from build123d import *

# Parameters (mm, degrees)
SKETCH2_R          = 1
CUT_EXTRUDE1_DEPTH = 52.147287318


with BuildPart() as part:
    # Sketch1 → Revolve1 (revolve)
    with BuildSketch(Plane.XY, mode=Mode.PRIVATE) as revolve1_sk:
        Polygon((32.65, -4.5), (10, -4.5), (10, -17.5), (7, -17.5), (7, 4.5), (32.65, 4.5), (32.65, 1.5), (28.65, 1.5), (28.65, -1.5), (32.65, -1.5), align=None)
    revolve(revolve1_sk.sketch.rotate(Axis((0, 0, 0), (0, 1, 0)), 90), axis=Axis((0, 0, 0), (0, 1, 0)))

    # Sketch2 → Cut-Extrude1 (cut, through all)
    with BuildSketch(Plane(origin=(0, 4.5, 0), x_dir=(1, 0, 0), z_dir=(0, 1, 0))):
        with Locations(Location((23.65, 0, 0), (0, 0, 270))):
            Circle(SKETCH2_R)
    extrude(amount=-CUT_EXTRUDE1_DEPTH, mode=Mode.SUBTRACT)


solid = part.part
The model under review builds one solid part; all positions refer to its coordinate system, in mm. A direction names the side the tool comes from. Coordinates: 2 decimals unless noted, no trailing zeros. Order: outer loops, then holes, each group sorted by start corner. A loop starts at its lowest first (then second) coordinate and runs counter-clockwise, first axis right, second up. Notation, with made-up numbers: (-8, 70.25) -> (48, 70.25) arc R37 ccw to (48, 106.25) -> close; hole circle Ø1 at (-39.75, 1). An arc over 180 degrees is marked (long way). Answer in a Markdown table with one row per item.
(1) Consider section C-C (y = -11). Write out the cut boundary in (x, z).
Answers:
| item | result |
|---|---|
| outline | circle Ø20 at (0, 0); hole circle Ø14 at (0, 0) |
(2) The part is to be moulded in two halves that separate along Y. For faces 1 (the flat face through (29, 1.5, 0)), 2 (the cylindrical face through (24.64, 0.06, -0.13)), 3 (the flat face through (29, -1.5, 0)), 4 (the flat face through (-8, 4.5, 0)), say which applies: +Y half, -Y half, draft (parallel to the pull), parting line (faces both ways), or undercut.
Answers:
| item | result |
|---|---|
| face 1 | undercut |
| face 2 | draft |
| face 3 | undercut |
| face 4 | +Y half |
(3) Consider section D-D (z = -22.5). Write out the cut boundary in (x, y), plus the area to 3 significant figures.
Answers:
| item | result |
|---|---|
| outline | (-23.66, -4.5) -> (23.66, -4.5) -> (23.66, -1.5) -> (17.74, -1.5) -> (17.74, 1.5) -> (23.66, 1.5) -> (23.66, 4.5) -> (-23.66, 4.5) -> (-23.66, 1.5) -> (-17.74, 1.5) -> (-17.74, -1.5) -> (-23.66, -1.5) -> close |
| area | 390 mm² |
(4) Wall thickness on line 1 along X through (y, z) = (-15.25, 0.5); line 2 along Y through (x, z) = (15.5, -6); line 3 along Y through (x, z) = (22.5, 18): over which ranges is each line inside the solid? List them lowest first.
Answers:
| item | result |
|---|---|
| line 1 | -9.99 to -6.98, 6.98 to 9.99 |
| line 2 | -4.5 to 4.5 |
| line 3 | -4.5 to -1.5, 1.5 to 4.5 |
(5) Insertion check: pin 1 (1.8 mm diameter, centred on x = 23.65, z = 0, fed in from +Y); pin 2 (2 mm diameter, centred on y = 1, z = -21, fed in from -X); pin 3 (5 mm diameter, centred on y = -1.5, z = -16.5, fed in from +X); pin 4 (3 mm diameter, centred on x = -8, y = -14, fed in from +Z). Each pin has a flat end and moves straight along its axis. Give the tip position at first contact, or say it passes through.
Answers:
| item | result |
|---|---|
| pin 1 | through |
| pin 2 | x = -25.7 |
| pin 3 | x = 29.5 |
| pin 4 | z = 7.6 |
(6) Consider section A-A (z = 0). Write out the cut boundary in (x, y), plus the area to 3 significant figures.
Answers:
| item | result |
|---|---|
| outline | (-32.65, -4.5) -> (-10, -4.5) -> (-10, -17.5) -> (-7, -17.5) -> (-7, 4.5) -> (-32.65, 4.5) -> (-32.65, 1.5) -> (-28.65, 1.5) -> (-28.65, -1.5) -> (-32.65, -1.5) -> close; (7, -17.5) -> (10, -17.5) -> (10, -4.5) -> (22.65, -4.5) -> (22.65, 4.5) -> (7, 4.5) -> close; (24.65, -4.5) -> (32.65, -4.5) -> (32.65, -1.5) -> (28.65, -1.5) -> (28.65, 1.5) -> (32.65, 1.5) -> (32.65, 4.5) -> (24.65, 4.5) -> close |
| area | 498 mm² |
(7) Consider section B-B (x = 0). Write out the cut boundary in (y, z).
Answers:
| item | result |
|---|---|
| outline | (-17.5, -10) -> (-4.5, -10) -> (-4.5, -32.65) -> (-1.5, -32.65) -> (-1.5, -28.65) -> (1.5, -28.65) -> (1.5, -32.65) -> (4.5, -32.65) -> (4.5, -7) -> (-17.5, -7) -> close; (-17.5, 7) -> (4.5, 7) -> (4.5, 32.65) -> (1.5, 32.65) -> (1.5, 28.65) -> (-1.5, 28.65) -> (-1.5, 32.65) -> (-4.5, 32.65) -> (-4.5, 10) -> (-17.5, 10) -> close |
(8) Machinability: for faces 5 (the cylindrical face through (0, -11, 10)), 6 (the cylindrical face through (-8.606, -0.021, -27.327)), 7 (the cylindrical face through (6.21, -6.35, -3.23)), which of the approach directions +Z, -Z, +X, -X, +Y, -Y give a long, thin tool a straight path to every point of the face, cutting with its end or side? Answer none if there is none.
Answers:
| item | result |
|---|---|
| face 5 | -Y |
| face 6 | none |
| face 7 | +Y, -Y |
